The model under review builds one solid part; all positions refer to its coordinate system, in mm. Round coordinates to 2 decimals unless told otherwise and drop trailing zeros. Write each loop counter-clockwise with the first axis right and the second up, starting at its lowest first coordinate (ties: lowest second). Pieces come first, ordered by that corner, then holes. Notation, with made-up numbers: (-40, 56.5) - (1, 56.5) arc R24 cw to (1, 83.5) - close; hole circle Ø7 at (61.5, -11.5). An arc over 180 degrees is marked (long way). Write each question's results on one line, items separated by ' | '.
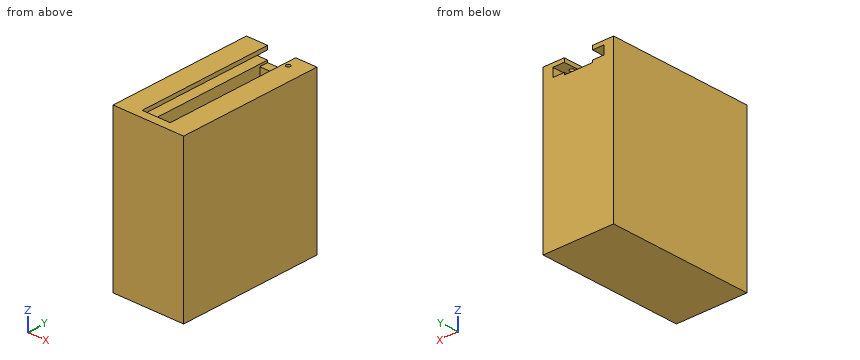
```python
from build123d import *

# Parameters (mm, degrees)
F0_W      = 6.6
F0_H      = 30
F1_DEPTH  = 2
F0_W_2    = 16.6
F0_H_2    = 34
F2_DEPTH  = 34
F3_R      = 1.5
F4_DEPTH  = 9
F5_W      = 6.6
F5_H      = 0.4
F6_DEPTH  = 25
F8_DEPTH  = 3
F9_W      = 12
F9_H      = 2
F10_DEPTH = 32
F11_R     = 0.5
F12_DEPTH = 4


with BuildPart() as f1:
    # F0 (on Top) → F1 (new body)
    with BuildSketch(Plane.XY):
        Rectangle(F0_W, F0_H)
    extrude(amount=F1_DEPTH)

    # F0 (on Top) → F2 (join)
    with BuildSketch(Plane.XY):
        Rectangle(F0_W_2, F0_H_2)
        Rectangle(F0_W, F0_H, mode=Mode.SUBTRACT)
    extrude(amount=F2_DEPTH)

    # F3 (on face) → F4 (join)
    with BuildSketch(Plane.XY.offset(2)):
        with Locations((0, 9)):
            Circle(F3_R)
        with Locations((0, -9)):
            Circle(F3_R)
    extrude(amount=F4_DEPTH)

    # F5 (on face) → F6 (cut)
    with BuildSketch(Plane(origin=(0, 17, 0), x_dir=(-1, 0, 0), z_dir=(0, 1, 0))):
        with Locations((0, 33.8)):
            Rectangle(F5_W, F5_H)
    extrude(amount=-F6_DEPTH, mode=Mode.SUBTRACT)

    # F7 (on face) → F8 (join)
    with BuildSketch(Plane.XY.offset(34)):
        Polygon((-8.3, -17), (8.3, -17), (8.3, 17), (3.3, 17), (3.3, -15), (-3.3, -15), (-3.3, 17), (-8.3, 17), align=None)
    extrude(amount=F8_DEPTH)

    # F9 (on face) → F10 (cut)
    with BuildSketch(Plane(origin=(0, 17, 0), x_dir=(-1, 0, 0), z_dir=(0, 1, 0))):
        with Locations((0, 35.1)):
            Rectangle(F9_W, F9_H)
    extrude(amount=-F10_DEPTH, mode=Mode.SUBTRACT)

    # F11 (on face) → F12 (cut)
    with BuildSketch(Plane.XY.offset(37)):
        with Locations((4.3, 14)):
            Circle(F11_R)
    extrude(amount=-F12_DEPTH, mode=Mode.SUBTRACT)


solid = f1.part
```
Q1. We need section D-D (z = 16). State the section outline as (x, y) points, plus the area to 3 significant figures.
Evaluation:
outline: (-8.3, -17) - (8.3, -17) - (8.3, 17) - (-8.3, 17) - close; hole (-3.3, -15) - (3.3, -15) - (3.3, 15) - (-3.3, 15) - close | area: 366 mm^2
Q2. Insertion check: P1, Ø0.6, axis at x = -1, y = 15.5, coming from the +Z side; P2, Ø0.5, axis at x = 4, y = 14, coming from the +Z side; P3, Ø1.5, axis at x = -0.5, y = -8.5, coming from the +Z side. Each pin has a flat end and moves straight along its axis. Give the tip position at first contact, or say it passes through.
Evaluation:
P1: stops at z = 33.6 | P2: stops at z = 37 | P3: stops at z = 11
Q3. For probe 1 along Y at (x, z) = (4.3, 33.55); probe 2 along Y at (x, z) = (0, 8.5); probe 3 along Y at (x, z) = (-1, 18), list the stretches that pass through material, from the lowest coordinate up.
Evaluation:
probe 1: y = -17 to 13.5, 14.5 to 17 | probe 2: y = -17 to -15, -10.5 to -7.5, 7.5 to 10.5, 15 to 17 | probe 3: y = -17 to -15, 15 to 17
Q4. We need section C-C (y = 0). State the section outline as (x, z) points, plus the area to 3 significant figures.
Evaluation:
outline: (-8.3, 0) - (8.3, 0) - (8.3, 37) - (3.3, 37) - (3.3, 36.1) - (6, 36.1) - (6, 34.1) - (3.3, 34.1) - (3.3, 2) - (-3.3, 2) - (-3.3, 34.1) - (-6, 34.1) - (-6, 36.1) - (-3.3, 36.1) - (-3.3, 37) - (-8.3, 37) - close | area: 372 mm^2
Q5. We need section B-B (x = 4.3). State the section outline as (y, z) points, plus the area to 3 significant figures.
Evaluation:
outline: (-17, 0) - (17, 0) - (17, 34.1) - (14.5, 34.1) - (14.5, 33) - (13.5, 33) - (13.5, 34.1) - (-15, 34.1) - (-15, 36.1) - (13.5, 36.1) - (13.5, 37) - (-17, 37) - close; (14.5, 36.1) - (17, 36.1) - (17, 37) - (14.5, 37) - close | area: 1,190 mm^2
Q6. We need section A-A (z = 2.5). State the section outline as (x, y) points, plus the area to 3 significant figures.
Evaluation:
outline: (-8.3, -17) - (8.3, -17) - (8.3, 17) - (-8.3, 17) - close; circle Ø3 at (0, -9); circle Ø3 at (0, 9); hole (-3.3, -15) - (3.3, -15) - (3.3, 15) - (-3.3, 15) - close | area: 381 mm^2
